Input: part model. Units: mm. Frame: model coordinates. A direction names the side the tool comes from. Round coordinates to 2 decimals unless told otherwise and drop trailing zeros. Loops run counter-clockwise (first coordinate to the right, second up) from the corner with the lowest first, then second, coordinate; pieces in that order, holes last. Notation, with made-up numbers: (80.5, -1.5) -> (138.5, -1.5) arc R21 ccw to (138.5, 16.5) -> close; hole circle Ø6 at (-19, 28). An arc over 180 degrees is marked (long way). One line per question, with ' | ' between items. Start each with the question number.
Q1. Access query for faces 1 (the face through (27.714, 62, -34)), 2 (the face through (-35.87, 62.77, 41.86)), 3 (the face through (-6, 102.5, 42)). Directions: +Z, -Z, +X, -X, +Y, -Y. A direction counts if a zero-diameter tool reaches every point of the face in a straight line with its end or side. Return the directions, or none.
Q2. Material intervals for L1, parallel to X at y = 100, z = 10; L2, parallel to Y at x = -14, z = 64; L3, parallel to Z at x = -27, y = 14, sorted ascending.
Q3. Cut plane B-B on y = 29.5. Return loops of the section in (x, z), and give its area (3 significant figures).
Q4. Cut plane A-A on z = 12. Return loops of the section in (x, y), and give its area (3 significant figures).
Q5. Mould query, pull axis X, two halves, no side actions, for faces 4 (the face through (40, 62, -66.012)), 5 (the face through (-18.85, 81.98, 59.7)), 6 (the face through (-126.882, 13.915, 11.663)), 7 (the face through (-147.286, 62, 11)). Classes: pulls with the +X half, pulls with the -X half, needs draft (parallel to the pull), parting line crosses it, or undercut.
Q6. Contact query for flat-ended pins moving along their axis: P1, Ø1, axis at x = -58, y = 61, coming from the -Z side; P2, Ø4, axis at y = 22.5, z = -19, coming from the -X side; P3, Ø3, axis at x = -104, y = 109.5, coming from the +Z side. Output: stop coordinate, or through.
Q7. Cut plane C-C on y = 59.5. Return loops of the section in (x, z), and give its area (3 significant figures).
Solid Edge part; units mm, degrees
sketch "Sketch1" plane through (0, 0, 0) normal (0, -1, 0) x (1, 0, 0)
  line L0 (-147.2861, 23.9877) -> (52.7139, 23.9877)
  line L1 (52.7139, 23.9877) -> (52.7139, -66.0123)
  line L2 (52.7139, -66.0123) -> (27.7139, -66.0123)
  line L3 (27.7139, -66.0123) -> (27.7139, -1.0123)
  line L4 (27.7139, -1.0123) -> (-147.2861, -1.0123)
  line L5 (-147.2861, -1.0123) -> (-147.2861, 23.9877)
extrude "Protrusion1" add sketch "Sketch1" against normal blind 125
sketch "Sketch2" plane through (84.5337, 62.5, -7.8321) normal (0.7071, 0, 0.7071) x (0, 1, 0)
  line L0 (-40, 45) -> (-40, 120)
  arc A0 (-40, 120) -> (40, 120) centre (0, 120) cw
  line L1 (40, 120) -> (40, 45)
extrude "Protrusion2" add sketch "Sketch2" against normal up to next material side at (26.1974, 22.55, 50.5042)
fillet "Round1" radius 25 4 edges at (-147.2861, 0, 11.4877) (40.2139, 0, -66.0123) (40.2139, 125, -66.0123) (-147.2861, 125, 11.4877)
hole "Hole1" at (52.7139, 25, -41.0123) direction (-1, 0, 0) diameter 24 end up to next
hole "Hole_2" at (52.7139, 100, -41.0123) direction (-1, 0, 0) diameter 24 end up to next
hole "Hole_3" at (-122.2861, 25, 23.9877) direction (0, 0, -1) diameter 24 end up to next
hole "Hole_4" at (-122.2861, 100, 23.9877) direction (0, 0, -1) diameter 24 end up to next
hole "Hole_5" at (-0.3191, 62.5, 77.0207) direction (-0.7071, 0, -0.7071) diameter 39 depth 50
sketch "Sketch3" plane through (-0.3191, 22.5, 50.5042) normal (0, -1, 0) x (1, 0, 0)
  line L0 (24.7487, 1.7678) -> (14.1421, -8.8388)
  line L1 (14.1421, -8.8388) -> (24.7487, -19.4454)
  line L2 (24.7487, -19.4454) -> (35.3553, -8.8388)
extrude "Cutout1" cut sketch "Sketch3" against normal through all material side at (19.1617, 22.5, 46.9333)
properties material "Steel"
Results:
1) face 1: -Z, -X, +Y, -Y | face 2: none | face 3: +Z, +X, -X, +Y
2) L1: -147.29 to -134.29, -110.29 to 52.71 | L2: 22.5 to 43.01, 81.99 to 102.5 | L3: -1.01 to 23.99
3) outline: (-147.29, -1.01) -> (-133.41, -1.01) -> (-133.41, 23.99) -> (-147.29, 23.99) -> close; (-111.16, -1.01) -> (27.71, -1.01) -> (27.71, -29.89) -> (52.71, -29.89) -> (52.71, 23.99) -> (35.04, 41.67) -> (24.43, 31.06) -> (13.82, 41.67) -> (24.43, 52.27) -> (-16.3, 93.01) -> (-85.32, 23.99) -> (-111.16, 23.99) -> close; (27.71, -66.01) -> (52.71, -66.01) -> (52.71, -52.14) -> (27.71, -52.14) -> close | area: 10,100 mm^2
4) outline: (-147.29, 25) arc R25 ccw to (-122.29, 0) -> (52.71, 0) -> (52.71, 125) -> (-122.29, 125) arc R25 ccw to (-147.29, 100) -> close; hole circle Ø24 at (-122.29, 25); hole circle Ø24 at (-122.29, 100) | area: 23,800 mm^2
5) face 4: needs draft | face 5: undercut | face 6: undercut | face 7: pulls with the -X half
6) P1: z = -1.01 | P2: x = 27.71 | P3: z = 23.99
7) outline: (-147.29, -1.01) -> (27.71, -1.01) -> (27.71, -66.01) -> (52.71, -66.01) -> (52.71, 23.99) -> (35.04, 41.67) -> (24.43, 31.06) -> (13.82, 41.67) -> (24.43, 52.27) -> (13.31, 63.4) -> (-22.05, 28.04) -> (-49.3, 55.29) -> (-13.94, 90.65) -> (-28.52, 105.23) -> (-109.76, 23.99) -> (-147.29, 23.99) -> close | area: 11,100 mm^2
